Part model, mm, in its own coordinate system. Round coordinates to 2 decimals unless told otherwise and drop trailing zeros. Write each loop counter-clockwise with the first axis right and the second up, starting at its lowest first coordinate (ties: lowest second). Pieces come first, ordered by that corner, then holes. Notation, with made-up numbers: M 54,83 L 95,83 A18 ccw 95,109 Z; hole C 51,14.5 d7. An arc over 180 degrees is marked long. One line per question, with ' | ' between items. Start each with the question number.
1) Saw through at C-C (y = -19.5). List the corners of the cut face in (x, z).
2) Saw through at B-B (x = -18.5). List the corners of the cut face in (y, z), plus the area to 3 significant figures.
3) Saw through at D-D (z = -21). List the corners of the cut face in (x, y), plus the area to 3 significant figures.
4) Saw through at A-A (z = 18). List the corners of the cut face in (x, y), plus the area to 3 significant figures.
5) Wall check: probe 1 along X at (y, z) = (-18, -24.5); probe 2 along Y at (x, z) = (27, -26); probe 3 along Y at (x, z) = (-26, -16). Give the ranges that are in metal, low to high. Write a range as [from, to].
```python
from build123d import *

# Parameters (mm, degrees)
SKETCH1_W            = 60
SKETCH1_H            = 60
BOSS_EXTRUDE1_DEPTH  = 30
LPATTERN2_COUNT      = 3
LPATTERN2_PITCH      = 15
LPATTERN2_COUNT_DIR2 = 3
LPATTERN2_PITCH_DIR2 = 15


with BuildPart() as part:
    # Sketch1 → Boss-Extrude1 (new body, symmetric)
    with BuildSketch(Plane.XY):
        Rectangle(SKETCH1_W, SKETCH1_H)
    extrude(amount=BOSS_EXTRUDE1_DEPTH, both=True)

    # Sketch3 → Cut-Revolve1 (revolve, cut)
    with BuildSketch(Plane(origin=(0, 0, 0), x_dir=(1, 0, 0), z_dir=(0, 1, 0))):
        with BuildLine():
            Line((0, -50), (62, -50))
            Line((62, -50), (62, 50))
            Line((62, 50), (0, 50))
            Line((0, 50), (0, 42.426406871))
            ThreePointArc((0, 42.426406871), (42.426406871, 0), (0, -42.426406871))
            Line((0, -42.426406871), (0, -50))
        make_face()
    revolve(axis=Axis((0, 0, -60.912631334), (0, 0, 1)), mode=Mode.SUBTRACT)

    # Sketch4 → Cut-Revolve2 (revolve, cut)
    with BuildSketch(Plane(origin=(0, 30, 0), x_dir=(1, 0, 0), z_dir=(0, 1, 0))):
        with BuildLine():
            Line((-15, -10), (-15, -20))
            ThreePointArc((-15, -20), (-10, -15), (-15, -10))
        make_face()
    cut_revolve2 = revolve(axis=Axis((-15, 30, 10), (0, 0, 1)), mode=Mode.SUBTRACT)

    # LPattern2: Cut-Revolve2 3 × 3, 4 skipped
    with Locations(*[(j * LPATTERN2_PITCH_DIR2, 0, -i * LPATTERN2_PITCH) for i in range(LPATTERN2_COUNT) for j in range(LPATTERN2_COUNT_DIR2) if (i, j) not in ((0, 0), (0, 1), (1, 0), (1, 2), (2, 1))]):
        add(cut_revolve2, mode=Mode.SUBTRACT)


solid = part.part
```
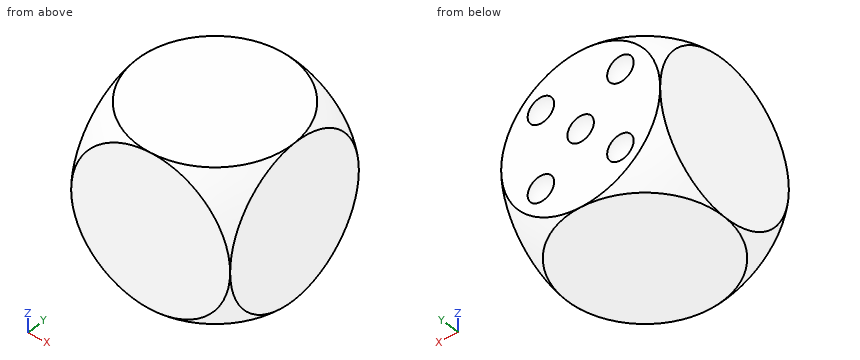
Answer key:
1) outline: M -30,-22.8 A37.68 ccw -22.8,-30 L 22.8,-30 A37.68 ccw 30,-22.8 L 30,22.8 A37.68 ccw 22.8,30 L -22.8,30 A37.68 ccw -30,22.8 Z
2) outline: M -30,-23.62 A38.18 ccw -23.62,-30 L 23.62,-30 A38.18 ccw 30,-23.62 L 30,-18.57 A3.57 cw 30,-11.43 L 30,11.43 A3.57 cw 30,18.57 L 30,23.62 A38.18 ccw 23.62,30 L -23.62,30 A38.18 ccw -30,23.62 Z | area: 3,480 mm2
3) outline: M -30,-21.42 A36.86 ccw -21.42,-30 L 21.42,-30 A36.86 ccw 30,-21.42 L 30,21.42 A36.86 ccw 21.42,30 L -21.42,30 A36.86 ccw -30,21.42 Z | area: 3,470 mm2
4) outline: M -30,-24 A38.42 ccw -24,-30 L 24,-30 A38.42 ccw 30,-24 L 30,24 A38.42 ccw 24,30 L 19,30 A4 cw 11,30 L -11,30 A4 cw -19,30 L -24,30 A38.42 ccw -30,24 Z | area: 3,480 mm2
5) probe 1: x = [-29.59, 29.59] | probe 2: y = [-19.87, 19.87] | probe 3: y = [-29.46, 29.46]
